Work out the finished part from the listing and answer in its coordinate system (mm). Face numbers are marked on the shaded views. A direction names the side the tool comes from. Give positions to 0.01 mm unless a question says otherwise; leave off trailing zeros. Loops run counter-clockwise (first coordinate to the right, second up) from the corner with the lowest first, then second, coordinate; pieces in that order, holes last. Notation, with made-up numbers: (-21, 31.25) - (1, 31.25) arc R18 ccw to (1, 61.25) - close; hole circle Ø4 at (45, -30.5). An arc over 180 degrees is marked (long way). One line per item, written item: value.
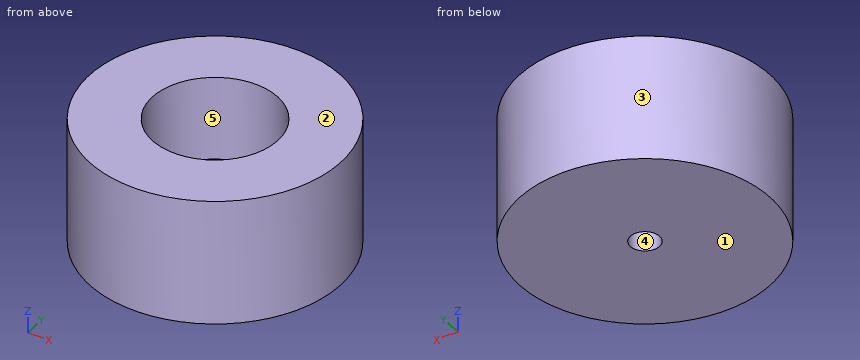
from build123d import *

# Parameters (mm, degrees)
SKETCH_R        = 15
PAD_DEPTH       = 15
SKETCH001_R     = 7.5
POCKET_DEPTH    = 10
SKETCH002_R     = 1.75
POCKET001_DEPTH = 10


with BuildPart() as part:
    # Sketch → Pad (new body)
    with BuildSketch(Plane.XY):
        Circle(SKETCH_R)
    extrude(amount=PAD_DEPTH)

    # Sketch001 (on Face3 of Pad) → Pocket (cut)
    with BuildSketch(Plane.XY.offset(15)):
        Circle(SKETCH001_R)
    extrude(amount=-POCKET_DEPTH, mode=Mode.SUBTRACT)

    # Sketch002 (on Face2 of Pocket) → Pocket001 (cut)
    with BuildSketch(Plane(origin=(0, 0, 0), x_dir=(1, 0, 0), z_dir=(0, 0, -1))):
        Circle(SKETCH002_R)
    extrude(amount=-POCKET001_DEPTH, mode=Mode.SUBTRACT)


solid = part.part
1. Find the intervals of material crossed by line 1 along Y through (x, z) = (0, 8.5); line 2 along Y through (x, z) = (0, 1.8); line 3 along Z through (x, y) = (0.5, -4), in increasing order.
Output:
line 1: y = -15 to -7.5, 7.5 to 15
line 2: y = -15 to -1.75, 1.75 to 15
line 3: z = 0 to 5
2. Section D-D (y = 6.5) is taken. Write down the section's boundary in (x, z), and give its area (3 significant figures).
Output:
outline: (-13.52, 0) - (13.52, 0) - (13.52, 15) - (3.74, 15) - (3.74, 5) - (-3.74, 5) - (-3.74, 15) - (-13.52, 15) - close
area: 331 mm²
3. For the marked faces 4 and 5, determine the directions among +Z, -Z, +X, -X, +Y, -Y from which every point of the face is accessible in a straight line to the end or side of a thin tool.
Output:
face 4: +Z, -Z
face 5: +Z
4. Section A-A (y = 0) is taken. Write down the section's boundary in (x, z).
Output:
outline: (-15, 0) - (-1.75, 0) - (-1.75, 5) - (-7.5, 5) - (-7.5, 15) - (-15, 15) - close; (1.75, 0) - (15, 0) - (15, 15) - (7.5, 15) - (7.5, 5) - (1.75, 5) - close
5. The mould has two halves that part along Z. Classify the marked faces 1, 2 and 3: released by +Z, released by -Z, zero draft, split by the parting line, or undercut.
Output:
face 1: released by -Z
face 2: released by +Z
face 3: zero draft
6. Section C-C (z = 4.5) is taken. Write down the section's boundary in (x, y).
Output:
outline: circle Ø30 at (0, 0); hole circle Ø3.5 at (0, 0)
7. Flat-ended cylindrical pins translate along their axes: pin 1 Ø1 at (y, z) = (10.5, 11.5) entering from +X; pin 2 Ø2 at (y, z) = (-2, 13.5) entering from +X; pin 3 Ø2 at (x, z) = (1.5, 7) entering from -Y. Find the tip coordinate at first contact, or state that the pin passes through.
Output:
pin 1: stops at x = 11.18
pin 2: stops at x = 14.97
pin 3: stops at y = -14.99
